```python
from build123d import *

# Parameters (mm, degrees)
SKETCH1_R                                       = 2
BOSS_EXTRUDE2_DEPTH                             = 3
CSK_FOR_M4_FLAT_HEAD_MACHINE_SCREW1_D           = 4.8
CSK_FOR_M4_FLAT_HEAD_MACHINE_SCREW1_DEPTH       = 22.23
CSK_FOR_M4_FLAT_HEAD_MACHINE_SCREW1_CSINK_D     = 9.4
CSK_FOR_M4_FLAT_HEAD_MACHINE_SCREW1_CSINK_ANGLE = 90
CSK_FOR_M4_FLAT_HEAD_MACHINE_SCREW1_TIP         = 1.442065486
CSK_FOR_M4_FLAT_HEAD_MACHINE_SCREW2_D           = 4.8
CSK_FOR_M4_FLAT_HEAD_MACHINE_SCREW2_DEPTH       = 22.23
CSK_FOR_M4_FLAT_HEAD_MACHINE_SCREW2_CSINK_D     = 9.4
CSK_FOR_M4_FLAT_HEAD_MACHINE_SCREW2_CSINK_ANGLE = 90
CSK_FOR_M4_FLAT_HEAD_MACHINE_SCREW2_TIP         = 1.442065486


with BuildPart() as part:
    # Sketch1 → Boss-Extrude2 (new body)
    with BuildSketch(Plane(origin=(0, 0, 0), x_dir=(1, 0, 0), z_dir=(0, 1, 0))):
        with BuildLine():
            Line((-28, 6), (0, 6))
            ThreePointArc((0, 6), (6, 0), (0, -6))
            Line((0, -6), (-28, -6))
            ThreePointArc((-28, -6), (-34, 0), (-28, 6))
        make_face()
        with Locations((-28, 0)):
            Circle(SKETCH1_R, mode=Mode.SUBTRACT)
        with Locations((-14, 0)):
            Circle(SKETCH1_R, mode=Mode.SUBTRACT)
        Circle(SKETCH1_R, mode=Mode.SUBTRACT)
    extrude(amount=BOSS_EXTRUDE2_DEPTH)

    # CSK for M4 Flat Head Machine Screw1
    with Locations(Plane(origin=(0, 3, 0), x_dir=(1, 0, 0), z_dir=(0, 1, 0))):
        with Locations((-14, 0)):
            CounterSinkHole(CSK_FOR_M4_FLAT_HEAD_MACHINE_SCREW1_D / 2, CSK_FOR_M4_FLAT_HEAD_MACHINE_SCREW1_CSINK_D / 2, depth=CSK_FOR_M4_FLAT_HEAD_MACHINE_SCREW1_DEPTH, counter_sink_angle=CSK_FOR_M4_FLAT_HEAD_MACHINE_SCREW1_CSINK_ANGLE)
            with Locations((0, 0, -(CSK_FOR_M4_FLAT_HEAD_MACHINE_SCREW1_DEPTH + CSK_FOR_M4_FLAT_HEAD_MACHINE_SCREW1_TIP / 2))):  # 118° drill point
                Cone(0, CSK_FOR_M4_FLAT_HEAD_MACHINE_SCREW1_D / 2, CSK_FOR_M4_FLAT_HEAD_MACHINE_SCREW1_TIP, mode=Mode.SUBTRACT)

    # CSK for M4 Flat Head Machine Screw2
    with Locations(Plane(origin=(0, 3, 0), x_dir=(1, 0, 0), z_dir=(0, 1, 0))):
        with Locations((-28, 0), (0, 0)):
            CounterSinkHole(CSK_FOR_M4_FLAT_HEAD_MACHINE_SCREW2_D / 2, CSK_FOR_M4_FLAT_HEAD_MACHINE_SCREW2_CSINK_D / 2, depth=CSK_FOR_M4_FLAT_HEAD_MACHINE_SCREW2_DEPTH, counter_sink_angle=CSK_FOR_M4_FLAT_HEAD_MACHINE_SCREW2_CSINK_ANGLE)
            with Locations((0, 0, -(CSK_FOR_M4_FLAT_HEAD_MACHINE_SCREW2_DEPTH + CSK_FOR_M4_FLAT_HEAD_MACHINE_SCREW2_TIP / 2))):  # 118° drill point
                Cone(0, CSK_FOR_M4_FLAT_HEAD_MACHINE_SCREW2_D / 2, CSK_FOR_M4_FLAT_HEAD_MACHINE_SCREW2_TIP, mode=Mode.SUBTRACT)


solid = part.part
```
Could you check a few things on this model? Use its own coordinates, in mm. Round coordinates to 2 decimals unless told otherwise and drop trailing zeros. Loops run counter-clockwise (first coordinate to the right, second up) from the corner with the lowest first, then second, coordinate; pieces in that order, holes last. Notation, with made-up numbers: (16, 65) - (25, 65) arc R6 ccw to (25, 70) - close; hole circle Ø1 at (35.25, 45). An arc over 180 degrees is marked (long way). Answer in a Markdown table with one row per item. Add a question column.
(1) If we mould it in two halves opening along X, with no side actions, what happens to faces 1 (the face through (6, 1, 0)), 2 (the face through (-9, 3, 0)), 3 (the face through (1.99, 0.81, 1.53)), 4 (the face through (-11.49, 0.81, -0.11))? For each: pulls with the +X half, pulls with the -X half, needs draft (parallel to the pull), parting line crosses it, or undercut.
(2) I need wall thicknesses on line 1 along Z through (x, y) = (-14, 0.45); line 2 along X through (y, z) = (0.2, -0.5); line 3 along X through (y, z) = (2.7, -2.5). Which ranges of each line are inside material? Lowest first, please.
(3) If we section it at C-C (y = 2): Please give me the cut outline in (x, z).
(4) If we section it at D-D (z = -2): State how many separate pieces and enclosed holes the cut face has, plus the area to 3 significant figures.
(5) If we section it at B-B (x = -14): Please give me the cut outline in (y, z).
(6) I'm going to push flat-ended pins straight in: pin 1 (4 mm diameter, centred on x = 0, z = 0, fed in from +Y); pin 2 (1 mm diameter, centred on x = -30, y = 2, fed in from -Z); pin 3 (6 mm diameter, centred on x = -14, z = 0, fed in from +Y). Where does each tip first touch, or does it pass through?
(7) If we section it at A-A (z = 0): Please give me the cut outline in (x, y), plus the area to 3 significant figures.
Model answer:
| question | item | result |
|---|---|---|
| 1 | face 1 | pulls with the +X half |
| 1 | face 2 | needs draft |
| 1 | face 3 | undercut |
| 1 | face 4 | undercut |
| 2 | line 1 | z = -6 to -2.4, 2.4 to 6 |
| 2 | line 2 | x = -33.98 to -30.35, -25.65 to -16.35, -11.65 to -2.35, 2.35 to 5.98 |
| 2 | line 3 | x = -33.45 to -31.62, -24.38 to -17.62, -10.38 to -3.62, 3.62 to 5.45 |
| 3 | outline | (-28, -6) - (0, -6) arc R6 ccw to (0, 6) - (-28, 6) arc R6 ccw to start; hole circle Ø7.4 at (-28, 0); hole circle Ø7.4 at (-14, 0); hole circle Ø7.4 at (0, 0) |
| 4 | separate pieces | 4 |
| 4 | enclosed holes | 0 |
| 4 | area | 72.5 mm² |
| 5 | outline | (0, -6) - (3, -6) - (3, -4.7) - (0.7, -2.4) - (0, -2.4) - close; (0, 2.4) - (0.7, 2.4) - (3, 4.7) - (3, 6) - (0, 6) - close |
| 6 | pin 1 | passes through |
| 6 | pin 2 | stops at z = -5.81 |
| 6 | pin 3 | stops at y = 1.3 |
| 7 | outline | (-34, 0) - (-30.4, 0) - (-30.4, 0.7) - (-32.7, 3) - (-34, 3) - close; (-25.6, 0) - (-16.4, 0) - (-16.4, 0.7) - (-18.7, 3) - (-23.3, 3) - (-25.6, 0.7) - close; (-11.6, 0) - (-2.4, 0) - (-2.4, 0.7) - (-4.7, 3) - (-9.3, 3) - (-11.6, 0.7) - close; (2.4, 0) - (6, 0) - (6, 3) - (4.7, 3) - (2.4, 0.7) - close |
| 7 | area | 60.9 mm² |
